from build123d import *

# Parameters (mm, degrees)
SKETCH009_W  = 5.019769
SKETCH009_H  = 1.561025
PAD007_DEPTH = 1
PAD005_DEPTH = 0.5
PAD006_DEPTH = 0.5
PAD008_DEPTH = 0.5
PAD009_DEPTH = 0.5


with BuildPart() as part:
    # Sketch009 → Pad007 (new body)
    with BuildSketch(Plane.XZ.offset(1.25)):
        with Locations((1.436677, 3.083954)):
            Rectangle(SKETCH009_W, SKETCH009_H)
    extrude(amount=PAD007_DEPTH)

    # Sketch005 → Pad005 (join)
    with BuildSketch(Plane(origin=(-0.75, 0, 0), x_dir=(0, 1, 0), z_dir=(0.996195, 0, 0.087156))):
        Polygon((-1.5, 3), (0.5, 3), (0.5, 17.5), (0, 17.5), (0, 3.5), (-1.5, 3.5), align=None)
    extrude(amount=PAD005_DEPTH)

    # Sketch006 → Pad006 (join)
    with BuildSketch(Plane(origin=(0.5, 0, 0), x_dir=(0, 1, 0), z_dir=(0.999391, 0, 0.034899))):
        Polygon((-1.5, 3), (0.5, 3), (0.5, 17.5), (0, 17.5), (0, 3.5), (-1.5, 3.5), align=None)
    extrude(amount=PAD006_DEPTH)

    # Sketch007 → Pad008 (join)
    with BuildSketch(Plane(origin=(1.75, 0, 0), x_dir=(0, 1, 0), z_dir=(0.999391, 0, -0.034899))):
        Polygon((-1.5, 3), (0.5, 3), (0.5, 17.5), (0, 17.5), (0, 3.5), (-1.5, 3.5), align=None)
    extrude(amount=PAD008_DEPTH)

    # Sketch008 → Pad009 (join)
    with BuildSketch(Plane(origin=(3, 0, 0), x_dir=(0, 1, 0), z_dir=(0.996195, 0, -0.087156))):
        Polygon((-1.5, 3), (0.5, 3), (0.5, 17.5), (0, 17.5), (0, 3.5), (-1.5, 3.5), align=None)
    extrude(amount=PAD009_DEPTH)


solid = part.part
The model under review builds one solid part; all positions refer to its coordinate system, in mm. Round coordinates to 2 decimals unless told otherwise and drop trailing zeros. Write each loop counter-clockwise with the first axis right and the second up, starting at its lowest first coordinate (ties: lowest second). Pieces come first, ordered by that corner, then holes. Notation, with made-up numbers: (30.25, 20) -> (72.25, 20) arc R29 ccw to (72.25, 52) -> close; hole circle Ø4 at (-23, 48.25). An arc over 180 degrees is marked (long way). Answer as a JSON object with one key per item and string values.
1. We need section D-D on x = 4.75. State the section outline as (y, z) points.
Results found:
{"outline": "(0, 14.27) -> (0.5, 14.27) -> (0.5, 17.41) -> (0, 17.41) -> close"}
2. The part is to be moulded in two halves that separate along X. For faces 1 (the face through (-1.6, 0.3, 9.7)), 2 (the face through (1, -2, 2.303)), 3 (the face through (3.85, 0.27, 9.71)), say which applies: pulls with the +X half, pulls with the -X half, needs draft (parallel to the pull), parting line crosses it, or undercut.
Results found:
{"face 1": "pulls with the -X half", "face 2": "needs draft", "face 3": "undercut"}
3. We need section B-B on z = 14.5. State the section outline as (x, y) points, and give its area (3 significant figures).
Results found:
{"outline": "(-2.02, 0) -> (-1.52, 0) -> (-1.52, 0.5) -> (-2.02, 0.5) -> close; (-0.01, 0) -> (0.49, 0) -> (0.49, 0.5) -> (-0.01, 0.5) -> close; (2.26, 0) -> (2.76, 0) -> (2.76, 0.5) -> (2.26, 0.5) -> close; (4.27, 0) -> (4.77, 0) -> (4.77, 0.5) -> (4.27, 0.5) -> close", "area": "1.00 mm^2"}
4. We need section A-A on y = -1. State the section outline as (x, z) points (3 decimals), and give its area (3 significant figures).
Results found:
{"outline": "(-1.055, 3.487) -> (-1.011, 2.989) -> (-0.513, 3.032) -> (-0.557, 3.53) -> close; (0.378, 3.498) -> (0.395, 2.998) -> (0.895, 3.016) -> (0.878, 3.515) -> close; (1.855, 2.998) -> (2.354, 2.981) -> (2.372, 3.48) -> (1.872, 3.498) -> close; (3.261, 2.989) -> (3.76, 2.945) -> (3.803, 3.443) -> (3.305, 3.487) -> close", "area": "1.00 mm^2"}
5. To check wall thickness, follow line 1 along X through (y, z) = (0.3, 15); line 2 along X through (y, z) = (0.15, 8); line 3 along Z through (x, y) = (-0.75, -2.05). State the ranges of each line that lie inside material, in increasing order.
Results found:
{"line 1": "x = -2.06 to -1.56, -0.02 to 0.48, 2.27 to 2.77, 4.31 to 4.81", "line 2": "x = -1.45 to -0.95, 0.22 to 0.72, 2.03 to 2.53, 3.7 to 4.2", "line 3": "z = 2.3 to 3.86"}
6. Clearance check with flat-ended pins moving along their axes: pin 1 (1.1 mm diameter, centred on x = 0.5, z = 13, fed in from -Y); pin 2 (3 mm diameter, centred on x = -1, z = 14, fed in from +Y); pin 3 (0.8 mm diameter, centred on y = -2, z = 3, fed in from -X); pin 4 (0.5 mm diameter, centred on y = -1.5, z = 3.5, fed in from +X). State where each tip first meets the part, or that it passes through.
Results found:
{"pin 1": "stops at y = 0", "pin 2": "stops at y = 0.5", "pin 3": "stops at x = -1.07", "pin 4": "stops at x = 3.95"}
7. We need section C-C on y = -1.6. State the section outline as (x, z) points.
Results found:
{"outline": "(-1.07, 2.3) -> (3.95, 2.3) -> (3.95, 3.86) -> (-1.07, 3.86) -> close"}
